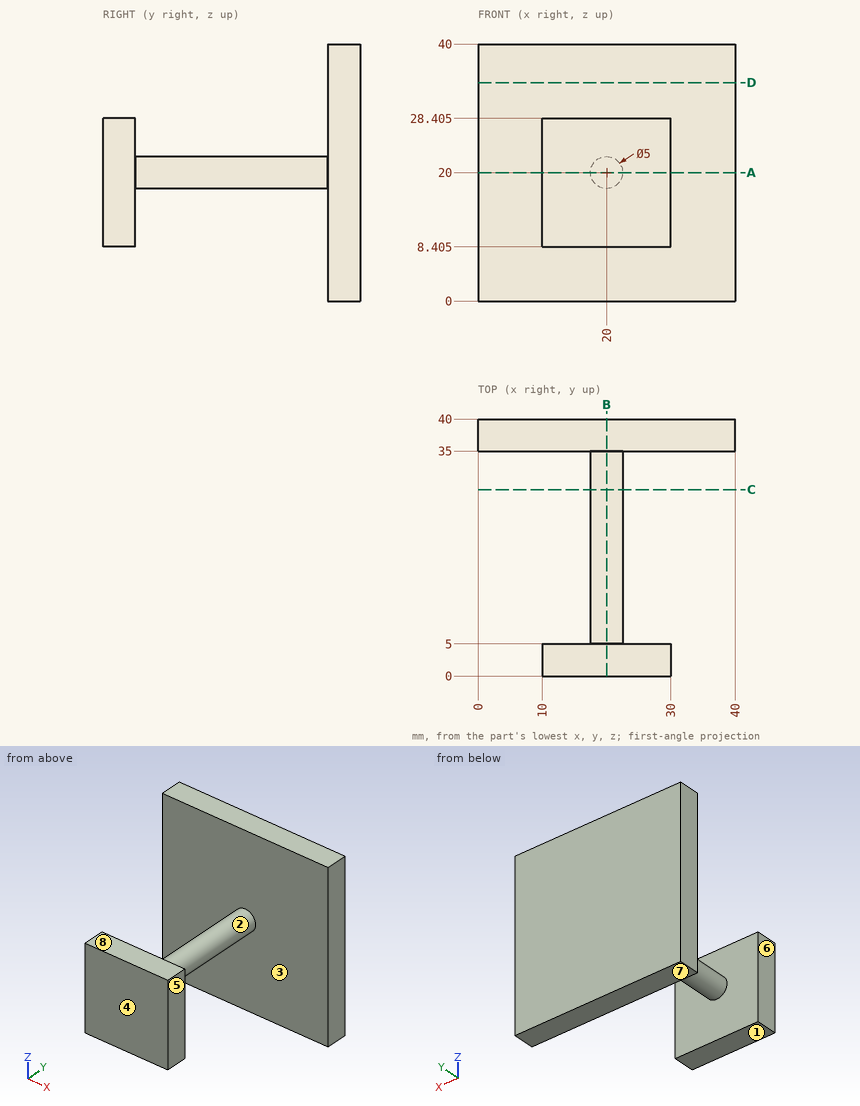
Input: dimensioned drawing with shaded views. Units: mm. Origin: part minimum x, y, z. A direction names the side the tool comes from. Round coordinates to 2 decimals unless told otherwise and drop trailing zeros. Loops run counter-clockwise (first coordinate to the right, second up) from the corner with the lowest first, then second, coordinate; pieces in that order, holes last. Notation, with made-up numbers: M -16,46.25 L -10,46.25 A24 ccw -10,60.25 Z; hole C -14,39.5 d5. An arc over 180 degrees is marked long. Answer in a Markdown table with one row per item. Add a question column.
1. Section B-B (x = 20). Output: boundary loops of the cut face in (y, z) (3 decimals).
2. Set-up query: the marked faces 5, 6, 7 and 8. Return all of +Z, -Z, +X, -X, +Y, -Y with unobstructed straight access to the full face (end or side cutting, diameter ignored); none if empty.
3. Ray query, probe 1 along Y at (x, z) = (29, 12); probe 2 along Y at (x, z) = (20, 33); probe 3 along X at (y, z) = (19, 21). Return the intervals inside material, ascending.
4. Section D-D (z = 34). Output: boundary loops of the cut face in (x, y).
5. Mould query, pull axis Y, two halves, no side actions, for the marked faces 1, 2, 3 and 4. Classes: released by +Y, released by -Y, zero draft, split by the parting line, or undercut.
6. Section C-C (y = 29). Output: boundary loops of the cut face in (x, z), and give its area (3 significant figures).
7. Section A-A (z = 20). Output: boundary loops of the cut face in (x, y), and give its area (3 significant figures).
8. Contact query for flat-ended pins moving along their axis: pin 1 (1.5 mm diameter, centred on y = 2.5, z = 14, fed in from -X); pin 2 (12 mm diameter, centred on y = 8, z = 15, fed in from +X); pin 3 (4 mm diameter, centred on x = 24, y = 3.5, fed in from +Z) (3 decimals). Output: stop coordinate, or through.
Values follow:
| question | item | result |
|---|---|---|
| 1 | outline | M 0,8.405 L 5,8.405 L 5,17.5 L 35,17.5 L 35,0 L 40,0 L 40,40 L 35,40 L 35,22.5 L 5,22.5 L 5,28.405 L 0,28.405 Z |
| 2 | face 5 | +Z, -Z, +X, -Y |
| 2 | face 6 | +Z, -Z, -X, -Y |
| 2 | face 7 | -Z, +X, -X, +Y, -Y |
| 2 | face 8 | +Z, +X, -X, -Y |
| 3 | probe 1 | 0 to 5, 35 to 40 |
| 3 | probe 2 | 35 to 40 |
| 3 | probe 3 | 17.71 to 22.29 |
| 4 | outline | M 0,35 L 40,35 L 40,40 L 0,40 Z |
| 5 | face 1 | zero draft |
| 5 | face 2 | undercut |
| 5 | face 3 | undercut |
| 5 | face 4 | released by -Y |
| 6 | outline | C 20,20 d5 |
| 6 | area | 19.6 mm^2 |
| 7 | outline | M 0,35 L 17.5,35 L 17.5,5 L 10,5 L 10,0 L 30,0 L 30,5 L 22.5,5 L 22.5,35 L 40,35 L 40,40 L 0,40 Z |
| 7 | area | 450 mm^2 |
| 8 | pin 1 | x = 10 |
| 8 | pin 2 | x = 30 |
| 8 | pin 3 | z = 28.405 |
